```python
from build123d import *

# Parameters (mm, degrees)
F1_DEPTH = 15
F2_R     = 0.74999
F3_R     = 1.25
F4_DEPTH = 8.2


# Not quite as in the source:
# - a fillet or chamfer is up to 0.001 mm smaller than in the source, because OpenCascade refuses the exact size


with BuildPart() as f1:
    # F0 (on Top) → F1 (new body)
    with BuildSketch(Plane.XY):
        with BuildLine():
            ThreePointArc((-3, 0), (2.1213203436, 2.1213203436), (0, -3))
            Line((0, -3), (-11, -3))
            Line((-11, -3), (-11, -4.5))
            Line((-11, -4.5), (0, -4.5))
            ThreePointArc((0, -4.5), (3.1819805153, 3.1819805153), (-4.5, 0))
            Line((-4.5, 0), (-4.5, -1))
            ThreePointArc((-4.5, -1), (-3.75, -1.75), (-3, -1))
            Line((-3, -1), (-3, 0))
        make_face()
    extrude(amount=F1_DEPTH)

    # F2 (radius 0.75 in the source; OpenCascade refuses exactly that, so slightly less here)
    f2_edges = [f1.edges().sort_by_distance(p)[0] for p in [
        (-11, -3, 7.5),
        (-11, -4.5, 7.5),
    ]]
    fillet(f2_edges, radius=F2_R)

    # F3 (on face) → F4 (cut)
    with BuildSketch(Plane(origin=(0, -3, 0), x_dir=(-1, 0, 0), z_dir=(0, 1, 0))):
        with Locations((8.25, 7.5)):
            Circle(F3_R)
    extrude(amount=-F4_DEPTH, mode=Mode.SUBTRACT)


solid = f1.part
```
For this review, take the finished solid that the model builds, in its own axes (mm). A direction names the side the tool comes from. Round coordinates to 2 decimals unless told otherwise and drop trailing zeros. Order: outer loops, then holes, each group sorted by start corner. A loop starts at its lowest first (then second) coordinate and runs counter-clockwise, first axis right, second up. Notation, with made-up numbers: (56, 70) -> (108, 70) arc R16 cw to (108, 82) -> close; hole circle Ø9 at (10, 54). An arc over 180 degrees is marked (long way). Use a Markdown table: item, result.
Item 1: Draft analysis for pull direction Y (two halves, no side actions). For faces 1 (the cylindrical face through (2.05, 2.19, 7.4)), 2 (the cylindrical face through (-7, -3.74, 7.55)), 3 (the cylindrical face through (3.285, 3.075, 7.395)), state which applies: +Y half, -Y half, draft (parallel to the pull), parting line (faces both ways), or undercut.
Resolved:
| item | result |
|---|---|
| face 1 | undercut |
| face 2 | draft |
| face 3 | parting line |
Item 2: Machinability: for faces 4 (the flat face through (-4.5, -0.5, 7.4)), 5 (the flat face through (-5, -3, 7)), 6 (the cylindrical face through (-3.77, -1.75, 7.4)), 7 (the flat face through (-3.3, -1, 15)), 8 (the flat face through (-5, -4.5, 7)), which of the approach directions +Z, -Z, +X, -X, +Y, -Y give a long, thin tool a straight path to every point of the face, cutting with its end or side? Answer none if there is none.
Resolved:
| item | result |
|---|---|
| face 4 | +Z, -Z, -X, +Y |
| face 5 | +Z, -Z, -X |
| face 6 | +Z, -Z |
| face 7 | +Z, +X, -X, +Y, -Y |
| face 8 | +Z, -Z, +X, -X, -Y |
Item 3: For line 1 along Y through (x, z) = (0, 5.5); line 2 along Z through (x, y) = (-8.25, -3.25); line 3 along Y through (x, z) = (-7.25, 12.5), list the stretches that pass through material, from the lowest coordinate up. Write a range as [from, to].
Resolved:
| item | result |
|---|---|
| line 1 | y = [-4.5, -3], [3, 4.5] |
| line 2 | z = [0, 6.25], [8.75, 15] |
| line 3 | y = [-4.5, -3] |
Item 4: Take a section at A-A (x = -8.25). State the section outline as (y, z) points, plus the area to 4 significant figures.
Resolved:
| item | result |
|---|---|
| outline | (-4.5, 0) -> (-3, 0) -> (-3, 6.25) -> (-4.5, 6.25) -> close; (-4.5, 8.75) -> (-3, 8.75) -> (-3, 15) -> (-4.5, 15) -> close |
| area | 18.75 mm² |
Item 5: For pin 1 (4 mm diameter, centred on y = 2.5, z = 12, fed in from -X); pin 2 (5 mm diameter, centred on x = 0, y = 0, fed in from +Z); pin 3 (3 mm diameter, centred on x = -5.5, z = 7.5, fed in from +Y), all flat-tipped, find the tip position at first contact; note any pin that passes through.
Resolved:
| item | result |
|---|---|
| pin 1 | stops at x = -4.47 |
| pin 2 | passes through |
| pin 3 | stops at y = 2.06 |
Item 6: Take a section at C-C (y = -1.5). State the section outline as (x, z) points.
Resolved:
| item | result |
|---|---|
| outline | (-4.31, 0) -> (-3.19, 0) -> (-3.19, 15) -> (-4.31, 15) -> close; (2.6, 0) -> (4.24, 0) -> (4.24, 15) -> (2.6, 15) -> close |
